Can you work these out from the model? Positions are in its coordinate system, mm. A direction names the side the tool comes from. Round coordinates to 2 decimals unless told otherwise and drop trailing zeros. Answer in a Markdown table with one row per item. Add a question column.
(1) If we mould it in two halves opening along Y, with no side actions, what happens to faces 5 (the face through (1.638, 0.968, 24.819)), 6 (the face through (5.8, 1.3, 12.3)), 7 (the face through (3, 0, 12))? For each: released by +Y, released by -Y, zero draft, split by the parting line, or undercut.
(2) If I drill on probe 1 along X at (y, z) = (1.2, 24); probe 2 along X at (y, z) = (1.8, 20.75); probe 3 along X at (y, z) = (0.2, 7.25), over which ranges is the centre line in solid material (lowest first)?
(3) For faces 1 (the face through (1.723, 1.051, 12.329)), 2 (the face through (1.641, 0.971, 0.185)), 3 (the face through (4.737, 0.943, 24.819)), 4 (the face through (0.6, 1.3, 12.3)), which set-ups out of +Z, -Z, +X, -X, +Y, -Y let a thin tool reach every point of the face, with its end or its side?
(4) I'm going to push flat-ended pins straight in: pin 1 (0.6 mm diameter, centred on x = 3, z = 12.5, fed in from +Y); pin 2 (1.5 mm diameter, centred on x = 4, z = 15.5, fed in from +Y); pin 3 (0.9 mm diameter, centred on y = 1.5, z = 13.5, fed in from +X). Where does each tip first touch, or does it pass through?
from build123d import *

# Parameters (mm, degrees)
F1_DEPTH    = 25
F2_T1_DEPTH = 25
F3_R        = 0.5
F4_T1_DEPTH = 26.7320508076
F5_R        = 0.2
F6_W        = 3.8095204468
F6_H        = 1.8
F7_DEPTH    = 25.0010001
F8_R        = 1.5
F9_SIZE     = 0.3


# Not quite as in the source:
# - a fillet or chamfer that OpenCascade refuses, or shapes differently, is made with other operations: its cross-section is extruded or revolved along the edge and cut away or added


with BuildPart() as f1:
    # F0 (on Top) → F1 (new body)
    with BuildSketch(Plane.XY):
        Polygon((0, 0.4), (0, 0), (6.4, 0), (6.4, 0.4), (5.8, 0.4), (5.8, 2.2), (6.1, 2.2), (6.1, 2.4), (0.3, 2.4), (0.3, 2.2), (0.6, 2.2), (0.6, 0.4), align=None)
    extrude(amount=F1_DEPTH)

    # F2: fillet of radius 0.5 on 2 edges, made by hand

    # F2_s2 → F2_t1 (join)
    with BuildSketch(Plane.XY):
        with BuildLine():
            ThreePointArc((0.3, 2.2), (0.5183300133, 2.0156037093), (0.6, 1.7417424305))
            Line((0.6, 1.7417424305), (0.6, 2.2))
            Line((0.6, 2.2), (0.3, 2.2))
        make_face()
        with BuildLine():
            ThreePointArc((5.8, 1.7417424305), (5.8816699867, 2.0156037093), (6.1, 2.2))
            Line((6.1, 2.2), (5.8, 2.2))
            Line((5.8, 2.2), (5.8, 1.7417424305))
        make_face()
    extrude(amount=F2_T1_DEPTH)

    # F3
    f3_edges = [f1.edges().sort_by_distance(p)[0] for p in [
        (5.8, 0.4, 12.5),
        (0.6, 0.4, 12.5),
    ]]
    fillet(f3_edges, radius=F3_R)

    # F4: fillet of radius 0.4 on 2 edges, made by hand

    # F4_s2 → F4_t1 (cut)
    with BuildSketch(Plane.XY.offset(-0.8660254038)):
        with BuildLine():
            ThreePointArc((0.3, 2.2), (0.4464101615, 2.3464101615), (0.6464101615, 2.4))
            Line((0.6464101615, 2.4), (0.3, 2.4))
            Line((0.3, 2.4), (0.3, 2.2))
        make_face()
        with BuildLine():
            ThreePointArc((5.7535898385, 2.4), (5.9535898385, 2.3464101615), (6.1, 2.2))
            Line((6.1, 2.2), (6.1, 2.4))
            Line((6.1, 2.4), (5.7535898385, 2.4))
        make_face()
    extrude(amount=F4_T1_DEPTH, mode=Mode.SUBTRACT)

    # F5
    f5_edges = [f1.edges().sort_by_distance(p)[0] for p in [
        (0.3, 2.2, 12.5),
        (6.1, 2.2, 12.5),
    ]]
    fillet(f5_edges, radius=F5_R)

    # F6 (on face) → F7 (cut, through all)
    with BuildSketch(Plane.XY.offset(25)):
        with Locations((3.2, 1.5)):
            Rectangle(F6_W, F6_H)
    extrude(amount=-F7_DEPTH, mode=Mode.SUBTRACT)

    # F8
    f8_edges = [f1.edges().sort_by_distance(p)[0] for p in [
        (1.29524, 0.6, 12.5),
        (5.10476, 0.6, 12.5),
    ]]
    fillet(f8_edges, radius=F8_R)

    # F9
    f9_edges = [f1.edges().sort_by_distance(p)[0] for p in [
        (3.2, 0.6, 25),
        (2.79524, 0.6, 12.5),
        (3.60476, 0.6, 12.5),
        (3.2, 0.6, 0),
        (6.4, 0, 12.5),
        (0, 0, 12.5),
        (1.29524, 2.25, 0),
        (1.73458, 1.03934, 0),
        (4.66542, 1.03934, 0),
        (5.10476, 2.25, 0),
        (1.29524, 2.25, 25),
        (1.73458, 1.03934, 25),
        (4.66542, 1.03934, 25),
        (5.10476, 2.25, 25),
    ]]
    chamfer(f9_edges, length=F9_SIZE)


solid = f1.part
Calculated:
| question | item | result |
|---|---|---|
| 1 | face 5 | released by +Y |
| 1 | face 6 | undercut |
| 1 | face 7 | released by -Y |
| 2 | probe 1 | 0.6 to 1.6, 4.8 to 5.8 |
| 2 | probe 2 | 0.6 to 1.33, 5.07 to 5.8 |
| 2 | probe 3 | 0.1 to 6.3 |
| 3 | face 1 | +Z, -Z, +Y |
| 3 | face 2 | -Z, +Y |
| 3 | face 3 | +Z, +Y |
| 3 | face 4 | +Z, -Z, -X |
| 4 | pin 1 | y = 0.6 |
| 4 | pin 2 | y = 1.13 |
| 4 | pin 3 | x = 5.85 |
